Input: part model. Units: mm. Frame: model coordinates. A direction names the side the tool comes from. Give positions to 0.01 mm unless a question says otherwise; leave off trailing zeros. Loops run counter-clockwise (first coordinate to the right, second up) from the corner with the lowest first, then second, coordinate; pieces in that order, holes last. Notation, with made-up numbers: (11, 82) - (52, 82) arc R8 ccw to (52, 86) - close; hole circle Ø4 at (-20, -40). An arc over 180 degrees is marked (long way). Answer as a JSON object with one key per item and string values.
from build123d import *

# Parameters (mm, degrees)
F0_W     = 50.8
F0_H     = 101.6
F0_W_2   = 44.45
F0_H_2   = 95.25
F1_DEPTH = 1786.7376
F2_R     = 2.54
F3_R     = 5.08


with BuildPart() as f1:
    # F0 (on Right) → F1 (new body)
    with BuildSketch(Plane.YZ):
        Rectangle(F0_W, F0_H)
        Rectangle(F0_W_2, F0_H_2, mode=Mode.SUBTRACT)
    extrude(amount=F1_DEPTH)

    # F2
    f2_edges = [f1.edges().sort_by_distance(p)[0] for p in [
        (893.3688, 22.225, 47.625),
        (893.3688, -22.225, 47.625),
        (893.3688, -22.225, -47.625),
        (893.3688, 22.225, -47.625),
    ]]
    fillet(f2_edges, radius=F2_R)

    # F3
    f3_edges = [f1.edges().sort_by_distance(p)[0] for p in [
        (893.3688, -25.4, -50.8),
        (893.3688, -25.4, 50.8),
        (893.3688, 25.4, 50.8),
        (893.3688, 25.4, -50.8),
    ]]
    fillet(f3_edges, radius=F3_R)


solid = f1.part
Item 1: Cut plane B-B (x = 946.5). Return loops of the section in (y, z) (3 decimals).
Geometry check:
{"outline": "(-25.4, -45.72) arc R5.08 ccw to (-20.32, -50.8) - (20.32, -50.8) arc R5.08 ccw to (25.4, -45.72) - (25.4, 45.72) arc R5.08 ccw to (20.32, 50.8) - (-20.32, 50.8) arc R5.08 ccw to (-25.4, 45.72) - close; hole (-22.225, -45.085) arc R2.54 ccw to (-19.685, -47.625) - (19.685, -47.625) arc R2.54 ccw to (22.225, -45.085) - (22.225, 45.085) arc R2.54 ccw to (19.685, 47.625) - (-19.685, 47.625) arc R2.54 ccw to (-22.225, 45.085) - close"}
Item 2: Cut plane C-C (y = 2). Return loops of the section in (x, z) (3 decimals).
Geometry check:
{"outline": "(0, -50.8) - (1786.738, -50.8) - (1786.738, -47.625) - (0, -47.625) - close; (0, 47.625) - (1786.738, 47.625) - (1786.738, 50.8) - (0, 50.8) - close"}
Item 3: Material intervals for line 1 (Z direction, x = 820, y = -13) (3 decimals); line 2 (Y direction, x = 983, z = 0) (3 decimals); line 3 (Z direction, x = 501, y = 21), sorted ascending. Write a range as [from, to].
Geometry check:
{"line 1": "z = [-50.8, -47.625], [47.625, 50.8]", "line 2": "y = [-25.4, -22.225], [22.225, 25.4]", "line 3": "z = [-50.75, -47.26], [47.26, 50.75]"}
Item 4: Mould query, pull axis Z, two halves, no side actions, for faces 1 (the face through (881, 0, 50.8)), 2 (the face through (881, -22.225, -1)), 3 (the face through (881, 0, 47.625)), 4 (the face through (881, 25.4, -1)). Classes: released by +Z, released by -Z, zero draft, split by the parting line, or undercut.
Geometry check:
{"face 1": "released by +Z", "face 2": "undercut", "face 3": "undercut", "face 4": "zero draft"}
Item 5: Cut plane A-A (z = -5.5). Return loops of the section in (x, y) (3 decimals), then the cut area to 3 significant figures.
Geometry check:
{"outline": "(0, -25.4) - (1786.738, -25.4) - (1786.738, -22.225) - (0, -22.225) - close; (0, 22.225) - (1786.738, 22.225) - (1786.738, 25.4) - (0, 25.4) - close", "area": "11,300 mm2"}
Item 6: Access query for faces 5 (the face through (881, 0, -47.625)), 6 (the face through (0, 22.5, 0.2)). Directions: +Z, -Z, +X, -X, +Y, -Y. A direction counts if a zero-diameter tool reaches every point of the face in a straight line with its end or side. Return the directions, or none.
Geometry check:
{"face 5": "+X, -X", "face 6": "+Z, -Z, -X, +Y, -Y"}
